from build123d import *

# Parameters (mm, degrees)
SKETCH1_R           = 14
BOSS_EXTRUDE1_DEPTH = 10
SKETCH3_R           = 3.263423297
CUT_EXTRUDE1_DEPTH  = 10
SKETCH4_R           = 1.5875
CUT_EXTRUDE2_DEPTH  = 133.522035903
LPATTERN1_COUNT     = 3
LPATTERN1_PITCH     = 38.1


with BuildPart() as part:
    # Sketch1 → Boss-Extrude1 (new body)
    with BuildSketch(Plane.XY):
        with BuildLine():
            Line((0, 16), (114.3, 16))
            ThreePointArc((114.3, 16), (130.3, 0), (114.3, -16))
            Line((114.3, -16), (0, -16))
            ThreePointArc((0, -16), (-16, 0), (0, 16))
        make_face()
        Circle(SKETCH1_R, mode=Mode.SUBTRACT)
        with Locations((38.1, 0)):
            Circle(SKETCH1_R, mode=Mode.SUBTRACT)
        with Locations((76.2, 0)):
            Circle(SKETCH1_R, mode=Mode.SUBTRACT)
        with Locations((114.3, 0)):
            Circle(SKETCH1_R, mode=Mode.SUBTRACT)
    extrude(amount=BOSS_EXTRUDE1_DEPTH)

    # Sketch3 → Cut-Extrude1 (cut)
    with BuildSketch(Plane(origin=(0, 16, 0), x_dir=(1, 0, 0), z_dir=(0, 1, 0))):
        with Locations(Location((19.05, -5, 0), (0, 0, 270))):
            Circle(SKETCH3_R)
    cut_extrude1 = extrude(amount=-CUT_EXTRUDE1_DEPTH, mode=Mode.SUBTRACT)

    # Sketch4 → Cut-Extrude2 (cut, through all)
    with BuildSketch(Plane(origin=(0, 6, 0), x_dir=(1, 0, 0), z_dir=(0, 1, 0))):
        with Locations(Location((19.05, -5, 0), (0, 0, 270))):
            Circle(SKETCH4_R)
    cut_extrude2 = extrude(amount=-CUT_EXTRUDE2_DEPTH, mode=Mode.SUBTRACT)

    # LPattern1: Cut-Extrude1, Cut-Extrude2 ×3
    with Locations(*[(i * LPATTERN1_PITCH, 0, 0) for i in range(1, LPATTERN1_COUNT)]):
        add(cut_extrude1, mode=Mode.SUBTRACT)
        add(cut_extrude2, mode=Mode.SUBTRACT)


solid = part.part
Here's how the part is built. I have some questions about the finished solid (model axes, mm). A direction names the side the tool comes from. Round coordinates to 2 decimals unless told otherwise and drop trailing zeros. Write each loop counter-clockwise with the first axis right and the second up, starting at its lowest first coordinate (ties: lowest second). Pieces come first, ordered by that corner, then holes. Notation, with made-up numbers: (35, -4.75) -> (61, -4.75) arc R21 cw to (61, 12.25) -> close; hole circle Ø4 at (65.5, 0). An arc over 180 degrees is marked (long way). One line per item, written item: value.
1) If I drill on line 1 (Z direction, x = 95.25, y = -5.5); line 2 (X direction, y = 9, z = 8.5); line 3 (Y direction, x = 115, z = 4), over which ranges is the centre line in solid material (lowest first)? Write a range as [from, to].
Filled sheet:
line 1: z = [0, 3.41], [6.59, 10]
line 2: x = [-13.23, -10.72], [10.72, 27.38], [48.82, 65.48], [86.92, 103.58], [125.02, 127.53]
line 3: y = [-15.98, -13.98], [13.98, 15.98]
2) I'm going to push flat-ended pins straight in: pin 1 Ø4 at (y, z) = (-7, 9) entering from -X; pin 2 Ø2 at (x, z) = (56.5, 4.5) entering from +Y; pin 3 Ø1.5 at (y, z) = (3, 6) entering from +X. Where does each tip first touch, or does it pass through?
Filled sheet:
pin 1: stops at x = -15.2
pin 2: stops at y = 6
pin 3: stops at x = 130.14
3) For faces 4 (the face through (98.486, 11.07, 4.575)), 5 (the face through (95.727, -4.846, 6.514)), which set-ups out of +Z, -Z, +X, -X, +Y, -Y let a thin tool reach every point of the face, with its end or its side?
Filled sheet:
face 4: +Y
face 5: +Y, -Y
4) Suppose I cut it at C-C on x = 38.1. List the corners of the cut face in (y, z) for me.
Filled sheet:
outline: (-16, 0) -> (-14, 0) -> (-14, 10) -> (-16, 10) -> close; (14, 0) -> (16, 0) -> (16, 10) -> (14, 10) -> close
5) We'd pull the mould along Z, two halves only. Please class faces 1 (the face through (53.964, 11.07, 4.293)), 2 (the face through (58, 0, 10)), 3 (the face through (89.55, 4.21, 4.93)): released by +Z, released by -Z, zero draft, split by the parting line, or undercut.
Filled sheet:
face 1: undercut
face 2: released by +Z
face 3: zero draft
6) Suppose I cut it at A-A on y = 0. Give the number of separate pieces and of enclosed holes in the cut face, plus the area to 3 significant figures.
Filled sheet:
separate pieces: 5
enclosed holes: 3
area: 319 mm2
